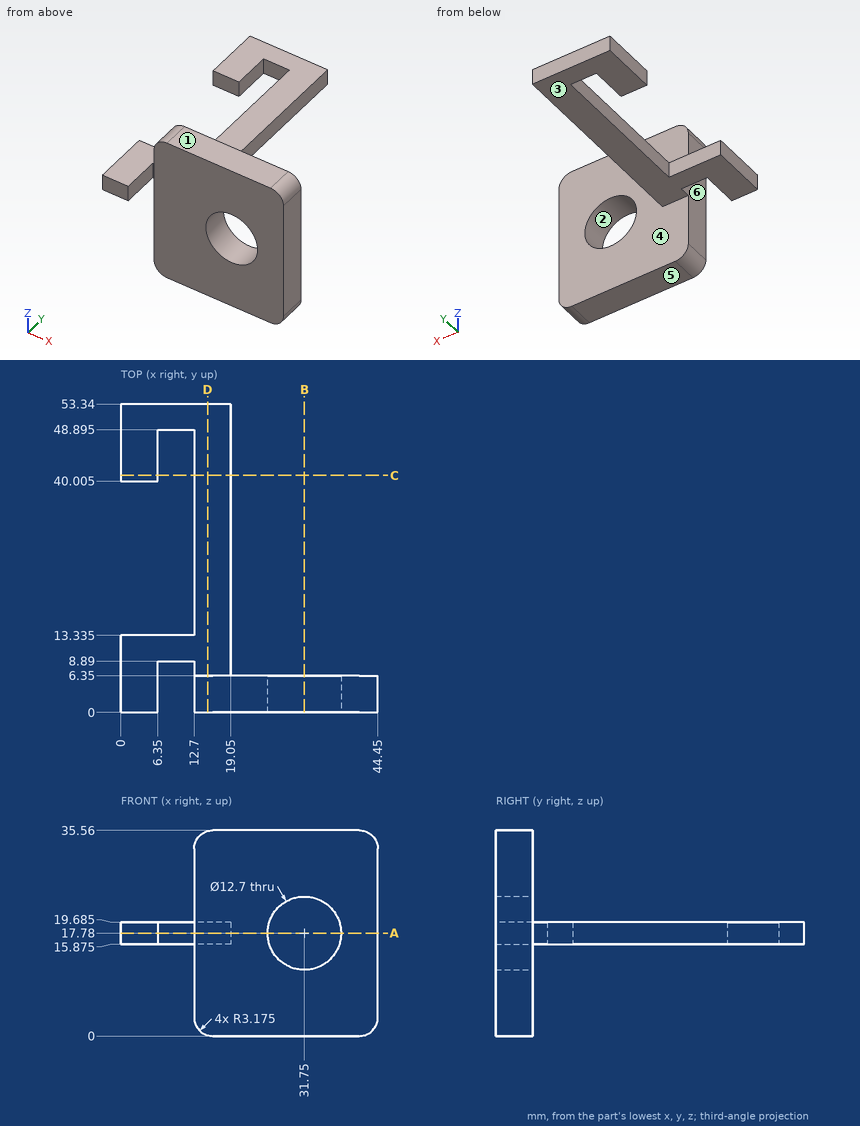
Check sheet for the drawn part. Datum: minimum x, y, z corner. Units: mm. A direction names the side the tool comes from. Round coordinates to 2 decimals unless told otherwise and drop trailing zeros. Order: outer loops, then holes, each group sorted by start corner. A loop starts at its lowest first (then second) coordinate and runs counter-clockwise, first axis right, second up. Notation, with made-up numbers: (59.25, -6) -> (112.25, -6) arc R34 cw to (112.25, 26) -> close; hole circle Ø1 at (70.25, -34.5). An arc over 180 degrees is marked (long way). Put each result on its own line as item: value. Start each with the question number.
(1) Material ranges on line 1 along X through (y, z) = (4, 17.78); line 2 along Z through (x, y) = (31.75, 4.5); line 3 along Y through (x, z) = (18.5, 28.5), recorded low to high.
(2) Section check A-A (z = 17.78). Enter the section's corners in (x, y) (3 decimals).
(3) Section check D-D (x = 15). Enter the section's corners in (y, z) (3 decimals), then the cut area to 3 significant figures.
(4) Tool access check on the marked faces 5 and 6. Record the directions out of +Z, -Z, +X, -X, +Y, -Y that give a thin tool (end or side, any length) a straight path to the whole face; none if there is none.
(5) Section check C-C (y = 41). Enter the section's corners in (x, z) (3 decimals).
(6) Draft check along Z on the marked faces 1, 2, 3 and 4. Enter one of: +Z half, -Z half, draft (parallel to the pull), parting line (faces both ways), or undercut.
(7) Section check B-B (x = 31.75). Enter the section's corners in (y, z), then the cut area to 3 significant figures.
(8) Depth check by flat-ended pin: pin 1 Ø3 at (y, z) = (33, 18) entering from +X; pin 2 Ø2.5 at (y, z) = (3, 24.5) entering from -X; pin 3 Ø4 at (x, z) = (28, 17) entering from +Y; pin 4 Ø5.5 at (x, y) = (7, 13.5) entering from -Z (3 decimals). Enter the tip coordinate at first touch or a pass-through.
Completed:
1. line 1: x = 0 to 6.35, 12.7 to 25.4, 38.1 to 44.45
1. line 2: z = 0 to 11.43, 24.13 to 35.56
1. line 3: y = 0 to 6.35
2. outline: (0, 0) -> (6.35, 0) -> (6.35, 8.89) -> (12.7, 8.89) -> (12.7, 0) -> (25.4, 0) -> (25.4, 6.35) -> (19.05, 6.35) -> (19.05, 53.34) -> (0, 53.34) -> (0, 40.005) -> (6.35, 40.005) -> (6.35, 48.895) -> (12.7, 48.895) -> (12.7, 13.335) -> (0, 13.335) -> close; (38.1, 0) -> (44.45, 0) -> (44.45, 6.35) -> (38.1, 6.35) -> close
3. outline: (0, 0.123) -> (6.35, 0.123) -> (6.35, 15.875) -> (53.34, 15.875) -> (53.34, 19.685) -> (6.35, 19.685) -> (6.35, 35.437) -> (0, 35.437) -> close
3. area: 403 mm2
4. face 5: -Z, +X, -X, +Y, -Y
4. face 6: +Z, -Z, -Y
5. outline: (0, 15.875) -> (6.35, 15.875) -> (6.35, 19.685) -> (0, 19.685) -> close; (12.7, 15.875) -> (19.05, 15.875) -> (19.05, 19.685) -> (12.7, 19.685) -> close
6. face 1: +Z half
6. face 2: undercut
6. face 3: -Z half
6. face 4: draft
7. outline: (0, 0) -> (6.35, 0) -> (6.35, 11.43) -> (0, 11.43) -> close; (0, 24.13) -> (6.35, 24.13) -> (6.35, 35.56) -> (0, 35.56) -> close
7. area: 145 mm2
8. pin 1: stops at x = 19.05
8. pin 2: stops at x = 12.7
8. pin 3: passes through
8. pin 4: stops at z = 15.875
